Job drawing, mm, ordinate dimensions from the low corner. One solid piece. Coordinates: 2 decimals unless noted, no trailing zeros. Loops run counter-clockwise (first coordinate to the right, second up) from the corner with the lowest first, then second, coordinate; pieces in that order, holes last. Notation, with made-up numbers: M 45.5,77 L 85.5,77 A6 cw 85.5,86 Z; hole C -40,-38.5 d6. An arc over 180 degrees is marked long. Answer as a JSON object with one key per item and string values. Group by question number.
1. Saw through at B-B on z = 2.5. Write the cut outline in (x, y), then the cut area to 3 significant figures.
2. Saw through at A-A on x = 3.5. Write the cut outline in (y, z), then the cut area to 4 significant figures.
3. Saw through at C-C on y = 44.5. Write the cut outline in (x, z), then the cut area to 3 significant figures.
4. Saw through at D-D on y = 20. Write the cut outline in (x, z), then the cut area to 3 significant figures.
5. Drill centre lines: L1, parallel to Y at x = 3.25, z = 5; L2, parallel to X at y = 3, z = 1.5; L3, parallel to Z at x = 3.75, y = 14.5. Where is each one in solid material? Low to high.
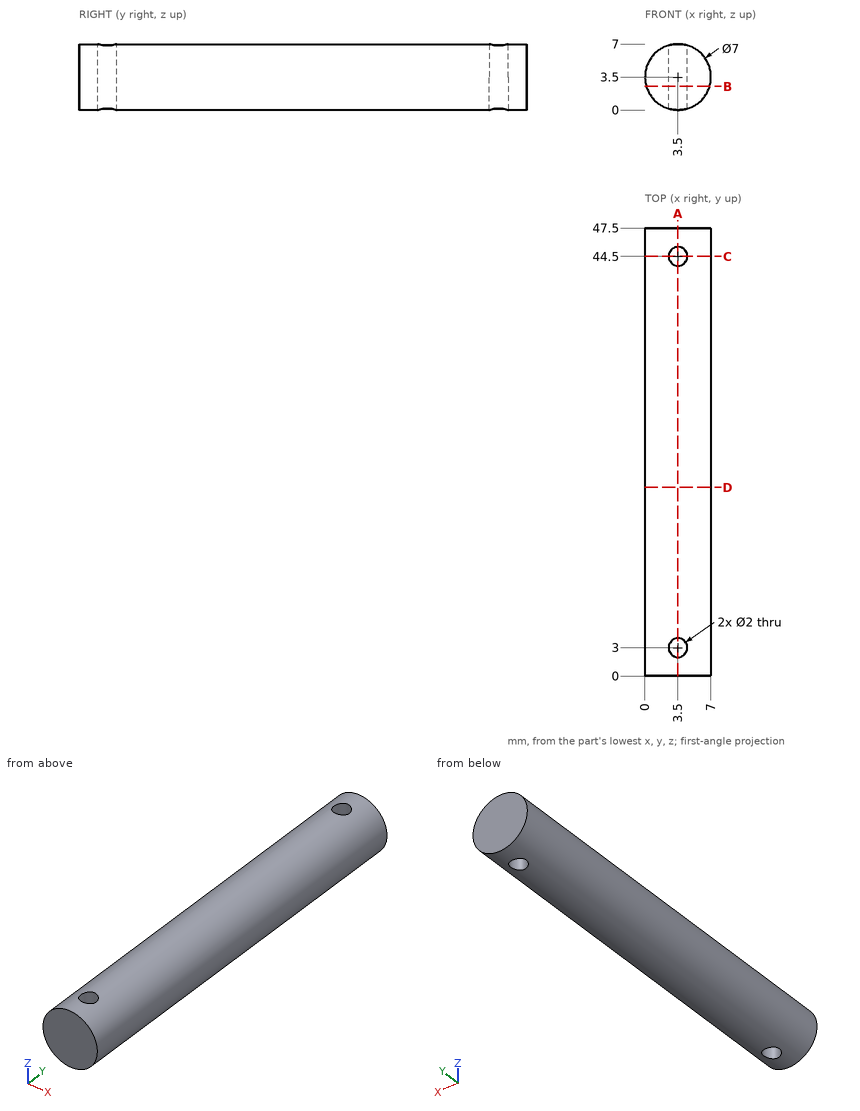
Outcome:
{
 "1": {"outline": "M 0.15,0 L 6.85,0 L 6.85,47.5 L 0.15,47.5 Z; hole C 3.5,3 d2; hole C 3.5,44.5 d2", "area": "312 mm²"},
 "2": {"outline": "M 0,0 L 2,0 L 2,7 L 0,7 Z; M 4,0 L 43.5,0 L 43.5,7 L 4,7 Z; M 45.5,0 L 47.5,0 L 47.5,7 L 45.5,7 Z", "area": "304.5 mm²"},
 "3": {"outline": "M 2.5,0.15 L 2.5,6.85 A3.5 ccw Z; M 4.5,0.15 A3.5 ccw 4.5,6.85 Z", "area": "24.7 mm²"},
 "4": {"outline": "C 3.5,3.5 d7", "area": "38.5 mm²"},
 "5": {"L1": "y = 0 to 2.03, 3.97 to 43.53, 45.47 to 47.5", "L2": "x = 0.63 to 2.5, 4.5 to 6.37", "L3": "z = 0.01 to 6.99"}
}
